Part model, mm, in its own coordinate system. Give positions to 0.01 mm unless a question says otherwise; leave off trailing zeros. Loops run counter-clockwise (first coordinate to the right, second up) from the corner with the lowest first, then second, coordinate; pieces in that order, holes last. Notation, with made-up numbers: M -12,-33 L 36,-33 A21 cw 36,6 Z; hole C 27,-18 d5. An arc over 180 degrees is marked long. Answer in a Markdown table with one row per item.
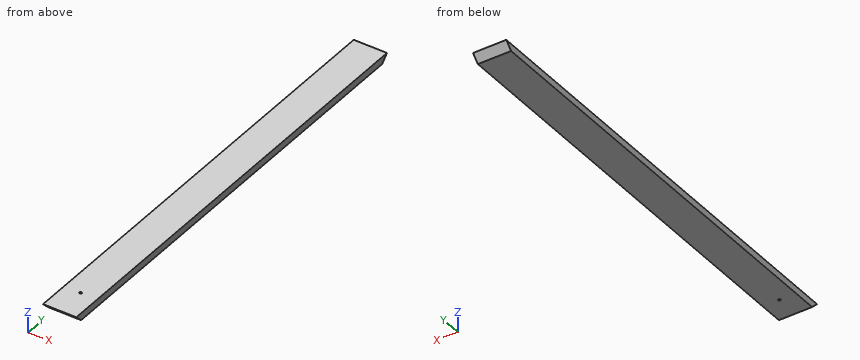
from build123d import *

# Parameters (mm, degrees)
F0_W     = 88.9
F0_H     = 19.05
F1_DEPTH = 1219.2
F3_DEPTH = 88.901
F5_D     = 6.35


with BuildPart() as f1:
    # F0 (on Front) → F1 (new body)
    with BuildSketch(Plane.XZ):
        Rectangle(F0_W, F0_H)
    extrude(amount=F1_DEPTH)

    # F2 (on face) → F3 (cut, through all)
    with BuildSketch(Plane.YZ.offset(44.45)):
        Polygon((0, -9.525), (0, 9.525), (-19.05, -9.525), align=None)
        Polygon((-1200.15, -9.525), (-1219.2, 9.525), (-1219.2, -9.525), align=None)
    extrude(amount=-F3_DEPTH, mode=Mode.SUBTRACT)

    # F5 (through all)
    with Locations(Plane.XY.offset(9.525)):
        with Locations((0, -1136.65)):
            Hole(F5_D / 2)


solid = f1.part
(1) Pin check, flat tips, straight feed: pin 1 Ø2 at (x, z) = (-22, -7.5) entering from -Y (3 decimals); pin 2 Ø2 at (x, z) = (19, 0) entering from -Y (3 decimals); pin 3 Ø8 at (x, z) = (0.5, 3.5) entering from +Y (3 decimals). Stop position of each tip, or through.
Recorded:
| item | result |
|---|---|
| pin 1 | stops at y = -1203.175 |
| pin 2 | stops at y = -1210.675 |
| pin 3 | stops at y = -2.025 |
(2) Saw through at A-A (x = 26). Write the cut outline in (y, z) (3 decimals), plus the area to 3 significant figures.
Recorded:
| item | result |
|---|---|
| outline | M -1219.2,9.525 L -1200.15,-9.525 L -19.05,-9.525 L 0,9.525 Z |
| area | 22,900 mm^2 |
(3) Drill centre lines: line 1 along X through (y, z) = (-1136.65, 3.5) (3 decimals); line 2 along Y through (x, z) = (-2, -4.5) (3 decimals); line 3 along Y through (x, z) = (0, -3.5) (3 decimals). Where is each one in solid material? Low to high.
Recorded:
| item | result |
|---|---|
| line 1 | x = -44.45 to -3.175, 3.175 to 44.45 |
| line 2 | y = -1205.175 to -1139.116, -1134.184 to -14.025 |
| line 3 | y = -1206.175 to -1139.825, -1133.475 to -13.025 |
